Job drawing, mm, ordinate dimensions from the low corner. One solid piece. Coordinates: 2 decimals unless noted, no trailing zeros. Order: outer loops, then holes, each group sorted by start corner. A loop starts at its lowest first (then second) coordinate and runs counter-clockwise, first axis right, second up. Notation, with made-up numbers: M -37,63 L -4,63 A15 cw -4,85 Z; hole C 61.5,24 d5. An arc over 180 degrees is marked long. Write item = value, one per line. Start each with the question number.
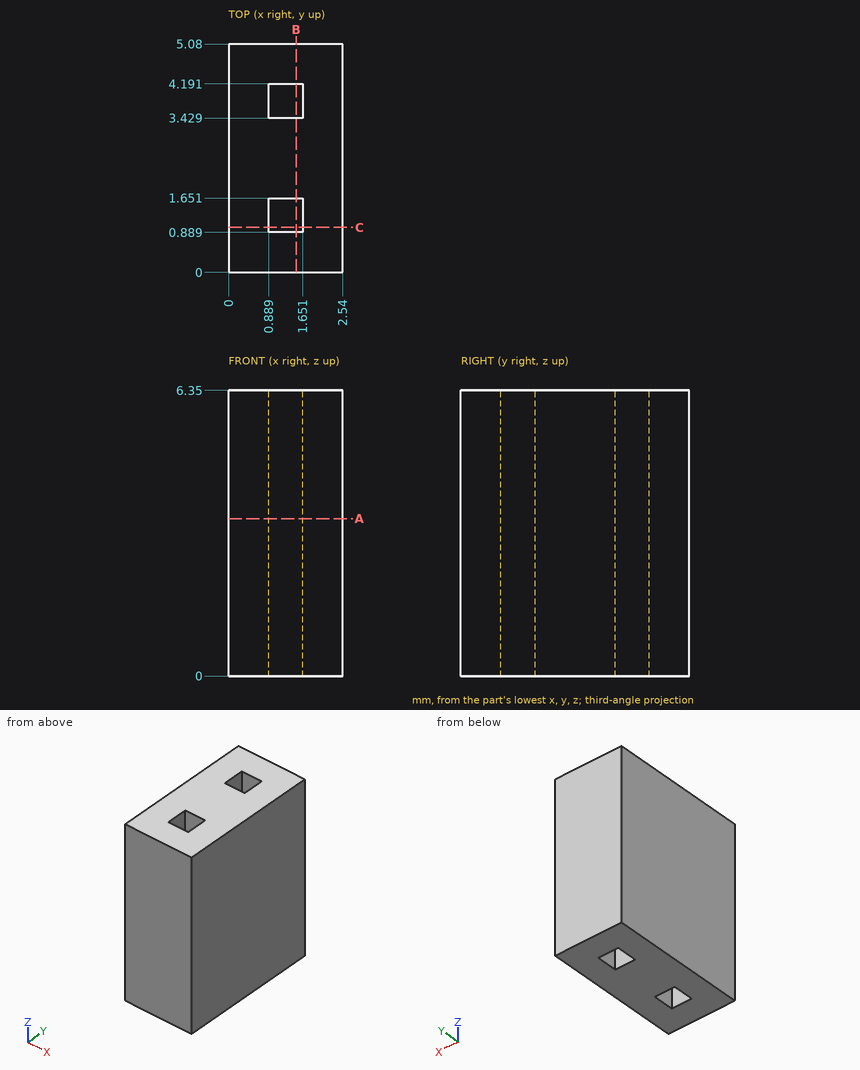
1. Slice it at B-B (x = 1.5). Write the cut outline in (y, z), plus the area to 3 significant figures.
2. Probe L1, parallel to Y at x = 1, z = 6.25; L2, parallel to X at y = 3.95, z = 6.25. List the from-to ranges inside material, lowest first.
3. Slice it at A-A (z = 3.5). Write the cut outline in (x, y), plus the area to 3 significant figures.
4. Slice it at C-C (y = 1). Write the cut outline in (x, z).
Calculated:
q1.outline = M 0,0 L 0.89,0 L 0.89,6.35 L 0,6.35 Z; M 1.65,0 L 3.43,0 L 3.43,6.35 L 1.65,6.35 Z; M 4.19,0 L 5.08,0 L 5.08,6.35 L 4.19,6.35 Z
q1.area = 22.6 mm²
q2.L1 = 0 to 0.89, 1.65 to 3.43, 4.19 to 5.08
q2.L2 = 0 to 0.89, 1.65 to 2.54
q3.outline = M 0,0 L 2.54,0 L 2.54,5.08 L 0,5.08 Z; hole M 0.89,0.89 L 1.65,0.89 L 1.65,1.65 L 0.89,1.65 Z; hole M 0.89,3.43 L 1.65,3.43 L 1.65,4.19 L 0.89,4.19 Z
q3.area = 11.7 mm²
q4.outline = M 0,0 L 0.89,0 L 0.89,6.35 L 0,6.35 Z; M 1.65,0 L 2.54,0 L 2.54,6.35 L 1.65,6.35 Z
